Answer from the drawing. Dimensions are ordinates in mm from the lowest x, y and z of the part. Round coordinates to 2 decimals unless told otherwise and drop trailing zeros. Loops run counter-clockwise (first coordinate to the right, second up) from the corner with the lowest first, then second, coordinate; pieces in that order, holes last.
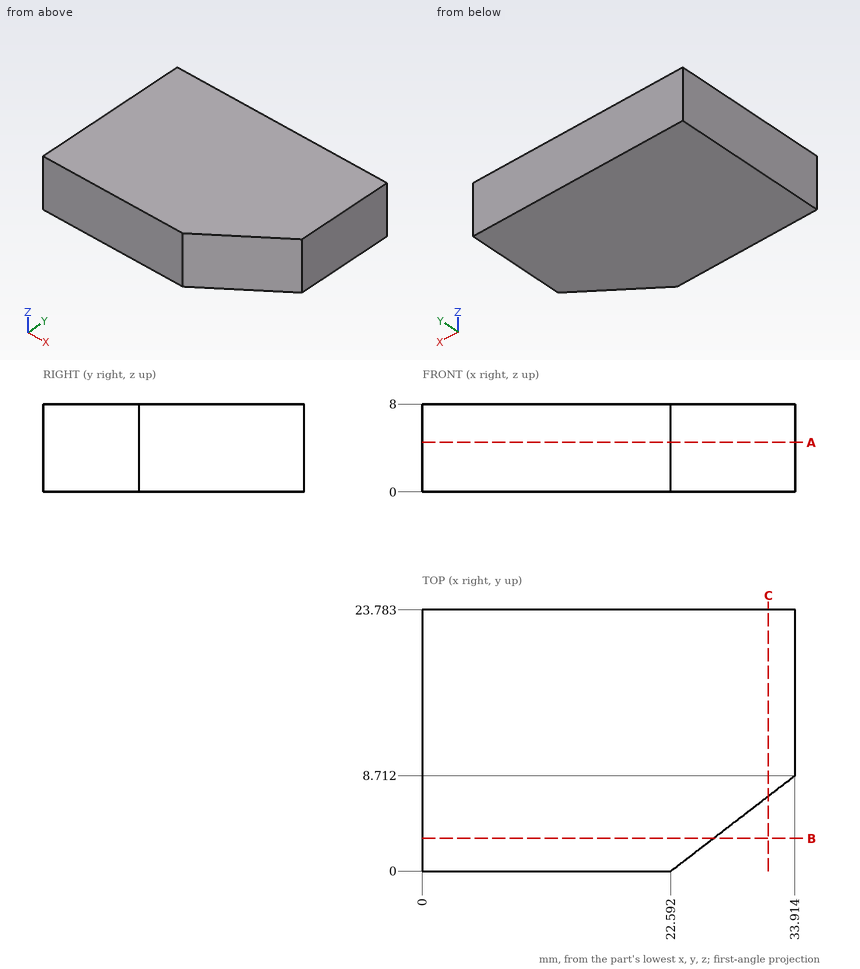
1. Consider probe 1 along X at (y, z) = (5.5, 3.5); probe 2 along Y at (x, z) = (29, 7.25); probe 3 along X at (y, z) = (4, 7.75). Determine where each line is inside the solid, lowest interval first.
Answer key:
probe 1: x = 0 to 29.74
probe 2: y = 4.93 to 23.78
probe 3: x = 0 to 27.79
2. Find section A-A (z = 4.5). Write down the section's boundary in (x, y), then the cut area to 3 significant figures.
Answer key:
outline: (0, 0) - (22.59, 0) - (33.91, 8.71) - (33.91, 23.78) - (0, 23.78) - close
area: 757 mm2
3. Find section C-C (x = 31.5). Write down the section's boundary in (y, z) (1 decimal).
Answer key:
outline: (6.9, 0) - (23.8, 0) - (23.8, 8) - (6.9, 8) - close
4. Find section B-B (y = 3). Write down the section's boundary in (x, z).
Answer key:
outline: (0, 0) - (26.49, 0) - (26.49, 8) - (0, 8) - close
